```python
from build123d import *

# Parameters (mm, degrees)
SKETCH_1_R          = 10
EXTRUDE_1_DEPTH     = 4.5
SKETCH_4_R          = 8
EXTRUDE_3_DEPTH     = 5
SKETCH_5_R          = 8
EXTRUDE_4_DEPTH     = 2.5
SKETCH_8_R          = 4
SKETCH_7_R          = 6
SKETCH_9_R          = 14.627232323
SKETCH_9_R_2        = 10
CUT_EXTRUDE_1_DEPTH = 18
SKETCH_10_R         = 2.5
CUT_EXTRUDE_2_DEPTH = 10
SKETCH_2_R          = 6
EXTRUDE_5_DEPTH     = 80
SKETCH_11_R         = 6
CUT_EXTRUDE_3_DEPTH = 36


with BuildPart() as part:
    # 草图1 → 凸台-拉伸1 (new body)
    with BuildSketch(Plane(origin=(0, 0, 0), x_dir=(1, 0, 0), z_dir=(0, 1, 0))):
        with Locations(Location((0, 0, 0), (0, 0, 270))):
            Circle(SKETCH_1_R)
    extrude(amount=EXTRUDE_1_DEPTH)

    # 草图4 → 凸台-拉伸3 (add, symmetric)
    with BuildSketch(Plane.XY):
        with BuildLine():
            Line((-10, 4.5), (10, 4.5))
            Line((10, 4.5), (10, 14.5))
            ThreePointArc((10, 14.5), (0, 24.5), (-10, 14.5))
            Line((-10, 14.5), (-10, 4.5))
        make_face()
        with Locations((0, 14.5)):
            Circle(SKETCH_4_R, mode=Mode.SUBTRACT)
    extrude(amount=EXTRUDE_3_DEPTH, both=True)

    # 草图5 → 凸台-拉伸4 (add, symmetric)
    with BuildSketch(Plane.XY):
        with Locations((0, 14.5)):
            Circle(SKETCH_5_R)
    extrude(amount=EXTRUDE_4_DEPTH, both=True)

    # 草图8 → 放样1 section 0
    with BuildSketch(Plane.XY.offset(4.5)):
        with Locations((0, 14.5)):
            Circle(SKETCH_8_R)
    # 草图7 → 放样1 section 1
    with BuildSketch(Plane.XY.offset(2.5)):
        with Locations((0, 14.5)):
            Circle(SKETCH_7_R)
    loft_1 = loft()

    # 镜向1: 放样1 across plane
    add(loft_1.mirror(Plane.XY))

    # 草图9 → 切除-拉伸1 (cut)
    with BuildSketch(Plane(origin=(0, 4.5, 0), x_dir=(1, 0, 0), z_dir=(0, 1, 0))):
        Circle(SKETCH_9_R)
        with Locations(Location((0, 0, 0), (0, 0, 150))):
            Circle(SKETCH_9_R_2, mode=Mode.SUBTRACT)
    extrude(amount=CUT_EXTRUDE_1_DEPTH, mode=Mode.SUBTRACT)

    # 草图10 → 切除-拉伸2 (cut)
    with BuildSketch(Plane.XY.offset(4.5)):
        with Locations((0, 14.5)):
            Circle(SKETCH_10_R)
    extrude(amount=-CUT_EXTRUDE_2_DEPTH, mode=Mode.SUBTRACT)

    # 草图2 → 凸台-拉伸5 (add)
    with BuildSketch(Plane.XZ):
        with Locations(Location((0, 0, 0), (0, 0, 270))):
            Circle(SKETCH_2_R)
    extrude(amount=EXTRUDE_5_DEPTH)

    # 草图11 → 切除-拉伸3 (cut)
    with BuildSketch(Plane.XY.offset(4.5)):
        with Locations((0, 14.5)):
            Circle(SKETCH_11_R)
    extrude(amount=-CUT_EXTRUDE_3_DEPTH, mode=Mode.SUBTRACT)

    # 草图12 → 切除-旋转1 (revolve, cut)
    with BuildSketch(Plane.XY):
        with BuildLine():
            Line((0, 8), (0, 21))
            ThreePointArc((0, 21), (6.5, 14.5), (0, 8))
        make_face()
    revolve(axis=Axis((0, 8, 0), (0, 1, 0)), mode=Mode.SUBTRACT)


solid = part.part
```
CAD build for the part. Positions are in the model's coordinates, mm. A direction names the side the tool comes from. Round coordinates to 2 decimals unless told otherwise and drop trailing zeros. Order: outer loops, then holes, each group sorted by start corner. A loop starts at its lowest first (then second) coordinate and runs counter-clockwise, first axis right, second up. Notation, with made-up numbers: (51.25, 63) - (96.25, 63) arc R11 ccw to (96.25, 83) - close; hole circle Ø1 at (-11.5, 85.5). An arc over 180 degrees is marked (long way). Use CSV: the item, a comma, the result in double quotes. Start each with the question number.
1) Two-plate mould, pull along X, no slides. Class faces 1 (the cylindrical face through (1.802, -39.44, -5.723)), 2 (the flat face through (0, -80, 0)), 3 (the cylindrical face through (-1.73, 6.69, -3.77)): pulls with the +X half, pulls with the -X half, needs draft (parallel to the pull), parting line crosses it, or undercut.
2) Tool access for faces 4 (the flat face through (0, 4.5, -7)), 5 (the cylindrical face through (-1.73, 6.69, 3.73)), 6 (the flat face through (3, 20, -2.5)), 7 (the flat face through (0, 6, 5)): list every direction of +Z, -Z, +X, -X, +Y, -Y with a clear straight run to the whole face (end or side of a thin tool).
3) Saw through at B-B (z = 1.5). List the corners of the cut face in (x, y), and give its area (3 significant figures).
4) Saw through at A-A (x = 0). List the corners of the cut face in (y, z), and give its area (3 significant figures).
5) Pin check, flat tips, straight feed: pin 1 Ø8 at (y, z) = (-14.5, 0.5) entering from -X; pin 2 Ø5 at (x, y) = (-1.5, 9.5) entering from +Z; pin 3 Ø12 at (x, y) = (-2, 1.5) entering from -Z; pin 4 Ø1.5 at (x, y) = (-3.5, -8.5) entering from -Z. Stop position of each tip, or through.
6) Saw through at C-C (y = 3). List the corners of the cut face in (x, z).
7) Wall check: L1, parallel to Y at x = 0, z = 4.5; L2, parallel to Y at x = -4, z = -8.5; L3, parallel to Y at x = 2.75, z = -4. Give the ranges that are in metal, low to high. Write a range as [from, to].
8) Saw through at D-D (z = -8.5). List the corners of the cut face in (x, y), and give its area (3 significant figures).
Values follow:
1,face 1,"parting line crosses it"
1,face 2,"needs draft"
1,face 3,"undercut"
2,face 4,"-Z, +X, -X, +Y"
2,face 5,"+Z"
2,face 6,"-Z"
2,face 7,"+Z, +X, -X, +Y"
3,outline,"(-9.89, 0) - (-5.81, 0) - (-5.81, -80) - (5.81, -80) - (5.81, 0) - (9.89, 0) - (9.89, 16) arc R10 ccw to (-9.89, 16) - close; hole circle Ø12.65 at (0, 14.5)"
3,area,"1,250 mm2"
4,outline,"(-80, -6) - (0, -6) - (0, -10) - (4.5, -10) - (4.5, -5) - (6.5, -5) - (6.5, -2.5) - (8.5, -2.5) arc R6.5 cw to (8.5, 2.5) - (6.5, 2.5) - (6.5, 5) - (4.5, 5) - (4.5, 10) - (0, 10) - (0, 6) - (-80, 6) - close; (20.5, -2.5) - (22.5, -2.5) - (22.5, -5) - (24.5, -5) - (24.5, 5) - (22.5, 5) - (22.5, 2.5) - (20.5, 2.5) arc R6.5 cw to start"
4,area,"1,110 mm2"
5,pin 1,"stops at x = -6"
5,pin 2,"stops at z = 2.5"
5,pin 3,"stops at z = -10"
5,pin 4,"stops at z = -5.33"
6,outline,"circle Ø20 at (0, 0)"
7,L1,"y = [-80, 6.5], [22.5, 24.5]"
7,L2,"y = [0, 4.5]"
7,L3,"y = [-80, 6.99], [22.01, 24.11]"
8,outline,"(-5.27, 0) - (5.27, 0) - (5.27, 4.5) - (-5.27, 4.5) - close"
8,area,"47.4 mm2"
